Part model, mm, in its own coordinate system. A direction names the side the tool comes from. Coordinates: 2 decimals unless noted, no trailing zeros. Order: outer loops, then holes, each group sorted by start corner. A loop starts at its lowest first (then second) coordinate and runs counter-clockwise, first axis right, second up.
1) Cut at A-A (y = 40.5). List the corners of the cut face in (x, z), and give its area (3 significant figures).
2) Wall check: L1, parallel to Y at x = -5.75, z = -10.5; L2, parallel to Y at x = -15.25, z = -4.5; L3, parallel to X at y = 9, z = -1. Give the ranges that are in metal, low to high.
3) Pin check, flat tips, straight feed: pin 1 Ø1.9 at (x, z) = (-14.5, -2) entering from +Y; pin 2 Ø8 at (x, z) = (-10, -8) entering from +Y; pin 3 Ø8 at (y, z) = (35, -1.5) entering from -X; pin 4 Ø12 at (x, y) = (-7, 35.5) entering from -Z. Stop position of each tip, or through.
4) Cut at B-B (y = 10.5). List the corners of the cut face in (x, z), and give its area (3 significant figures).
5) Tool access for faces 1 (the cylindrical face through (-25.003, 14.544, -0.941)), 2 (the cylindrical face through (-15.083, 31.24, -5.082)): list every direction of +Z, -Z, +X, -X, +Y, -Y with a clear straight run to the whole face (end or side of a thin tool).
```python
from build123d import *

# Parameters (mm, degrees)
SKETCH1_R           = 12
BOSS_EXTRUDE1_DEPTH = 30.5
SKETCH1_3_R         = 3.25
SKETCH1_3_R_2       = 1
BOSS_EXTRUDE2_DEPTH = 32
SKETCH1_4_R         = 1
BOSS_EXTRUDE3_DEPTH = 44.5
FILLET1_R           = 0.5
FILLET2_R           = 1


with BuildPart() as part:
    # Sketch1 → Boss-Extrude1 (new body)
    with BuildSketch(Plane(origin=(0, 0, 0), x_dir=(1, 0, 0), z_dir=(0, 1, 0))):
        with Locations(Location((-13.105100699, 2.502858666, 0), (0, 0, 90))):
            Circle(SKETCH1_R)
    extrude(amount=BOSS_EXTRUDE1_DEPTH)

    # Sketch1_3 → Boss-Extrude2 (add)
    with BuildSketch(Plane(origin=(0, 0, 0), x_dir=(1, 0, 0), z_dir=(0, 1, 0))):
        with Locations(Location((-13.105100699, 2.502858666, 0), (0, 0, 270))):
            Circle(SKETCH1_3_R)
        with Locations(Location((-13.105100699, 2.502858666, 0), (0, 0, 270))):
            Circle(SKETCH1_3_R_2, mode=Mode.SUBTRACT)
    extrude(amount=BOSS_EXTRUDE2_DEPTH)

    # Sketch1_4 → Boss-Extrude3 (add)
    with BuildSketch(Plane(origin=(0, 0, 0), x_dir=(1, 0, 0), z_dir=(0, 1, 0))):
        with Locations(Location((-13.105100699, 2.502858666, 0), (0, 0, 270))):
            Circle(SKETCH1_4_R)
    extrude(amount=BOSS_EXTRUDE3_DEPTH)

    # Fillet1
    fillet1_edges = [part.edges().sort_by_distance(p)[0] for p in [
        (-13.105100699, 44.5, -3.502858666),
    ]]
    fillet(fillet1_edges, radius=FILLET1_R)

    # Fillet2
    fillet2_edges = [part.edges().sort_by_distance(p)[0] for p in [
        (-13.105100699, 30.5, 9.497141334),
    ]]
    fillet(fillet2_edges, radius=FILLET2_R)


solid = part.part
```
Geometry check:
1. outline: circle Ø2 at (-13.11, -2.5)
1. area: 3.14 mm2
2. L1: y = 0 to 30.5
2. L2: y = 0 to 32
2. L3: x = -25.01 to -1.2
3. pin 1: stops at y = 44.5
3. pin 2: stops at y = 32
3. pin 3: stops at x = -16.36
3. pin 4: stops at z = -13.78
4. outline: circle Ø24 at (-13.11, -2.5)
4. area: 452 mm2
5. face 1: +Y, -Y
5. face 2: +Y
